For this review, take the finished solid that the model builds, in its own axes (mm). A direction names the side the tool comes from. Round coordinates to 2 decimals unless told otherwise and drop trailing zeros. Order: outer loops, then holes, each group sorted by start corner. A loop starts at its lowest first (then second) coordinate and runs counter-clockwise, first axis right, second up. Notation, with made-up numbers: (55, -12) -> (75, -12) arc R24 ccw to (75, 1) -> close; hole circle Ø1 at (85.25, 0). An arc over 180 degrees is marked (long way). Answer in a Markdown table with one row per item.
```python
from build123d import *

# Parameters (mm, degrees)
SKETCH_1_R               = 30
SKETCH_1_R_2             = 28.6
EXTRUDE_1_DEPTH          = 64
PATTERN_CIRCULAR_1_COUNT = 8
SKETCH_10_W              = 100
SKETCH_10_H              = 100
SKETCH_10_R              = 1.8
SKETCH_10_R_2            = 28.559863413
EXTRUDE_2_DEPTH          = 10


with BuildPart() as part:
    # 스케치1 → 보스-돌출1 (new body)
    with BuildSketch(Plane(origin=(0, 0, 0), x_dir=(1, 0, 0), z_dir=(0, 1, 0))):
        with Locations(Location((0, 0, 0), (0, 0, 270))):
            Circle(SKETCH_1_R)
        with Locations(Location((0, 0, 0), (0, 0, 270))):
            Circle(SKETCH_1_R_2, mode=Mode.SUBTRACT)
    extrude(amount=EXTRUDE_1_DEPTH)

    # 스케치9 → M2 남비 머리 나사용 카운터보어1 (revolve, cut)
    with BuildSketch(Plane(origin=(-30, 5, 0), x_dir=(0, 0, 1), z_dir=(0, 1, 0))):
        Polygon((0, 0), (0, 10.721032743), (1.2, 10), (1.2, 1), (2.5, 1), (2.5, 0), align=None)
    hole_wizard_m2_1 = revolve(axis=Axis((-36.35, 5, 0), (1, 0, 0)), mode=Mode.SUBTRACT)

    # 원형 패턴1: M2 남비 머리 나사용 카운터보어1 ×8 about axis
    pattern_circular_1_axis = Axis((0, 0, 0), (0, 1, 0))
    for i in range(1, PATTERN_CIRCULAR_1_COUNT):
        add(hole_wizard_m2_1.rotate(pattern_circular_1_axis, i * 360 / PATTERN_CIRCULAR_1_COUNT), mode=Mode.SUBTRACT)

    # 스케치10 → 보스-돌출2 (add)
    with BuildSketch(Plane(origin=(0, 64, 0), x_dir=(1, 0, 0), z_dir=(0, 1, 0))):
        Rectangle(SKETCH_10_W, SKETCH_10_H)
        with Locations(Location((41.7, -41.7, 0), (0, 0, 270))):
            Circle(SKETCH_10_R, mode=Mode.SUBTRACT)
        with Locations(Location((41.7, 41.7, 0), (0, 0, 270))):
            Circle(SKETCH_10_R, mode=Mode.SUBTRACT)
        with Locations(Location((-41.7, 41.7, 0), (0, 0, 270))):
            Circle(SKETCH_10_R, mode=Mode.SUBTRACT)
        with Locations(Location((-41.7, -41.7, 0), (0, 0, 270))):
            Circle(SKETCH_10_R, mode=Mode.SUBTRACT)
        with Locations(Location((0, 0, 0), (0, 0, 270))):
            Circle(SKETCH_10_R_2, mode=Mode.SUBTRACT)
    extrude(amount=EXTRUDE_2_DEPTH)


solid = part.part
```
Q1. Clearance check with flat-ended pins moving along their axes: pin 1 Ø4 at (x, y) = (0, 5) entering from +Z; pin 2 Ø4 at (x, y) = (0, 5) entering from -Z; pin 3 Ø2 at (x, y) = (-3, 13.5) entering from +Z; pin 4 Ø4.5 at (x, z) = (41.7, 41.7) entering from +Y. State where each tip first meets the part, or that it passes through.
Answer key:
| item | result |
|---|---|
| pin 1 | stops at z = 29 |
| pin 2 | stops at z = -29 |
| pin 3 | stops at z = 29.93 |
| pin 4 | stops at y = 74 |
Q2. Take a section at D-D, the plane x = -6.5. Write out the cut boundary in (y, z).
Answer key:
| item | result |
|---|---|
| outline | (0, -29.29) -> (64, -29.29) -> (64, -50) -> (74, -50) -> (74, -27.81) -> (64, -27.81) -> (64, -27.85) -> (0, -27.85) -> close; (0, 27.85) -> (64, 27.85) -> (64, 27.81) -> (74, 27.81) -> (74, 50) -> (64, 50) -> (64, 29.29) -> (0, 29.29) -> close |
Q3. Take a section at C-C, the plane z = -11.5. Write out the cut boundary in (x, y).
Answer key:
| item | result |
|---|---|
| outline | (-50, 64) -> (-27.71, 64) -> (-27.71, 0) -> (-26.19, 0) -> (-26.19, 64) -> (-26.14, 64) -> (-26.14, 74) -> (-50, 74) -> close; (26.14, 64) -> (26.19, 64) -> (26.19, 0) -> (27.71, 0) -> (27.71, 64) -> (50, 64) -> (50, 74) -> (26.14, 74) -> close |
Q4. Tool access review of faces 4 (the face through (-29, 4, -1)), 5 (the face through (-1, 6, -29)), 6 (the face through (22.55, 4.25, 19.18)), 7 (the face through (-11.49, 31.552, 27.712)), 8 (the face through (-1, 69, -50)): name each direction out of +Z, -Z, +X, -X, +Y, -Y from which nothing blocks a thin tool from reaching the whole face with its end or side.
Answer key:
| item | result |
|---|---|
| face 4 | -X |
| face 5 | -Z |
| face 6 | none |
| face 7 | -Y |
| face 8 | -Z, +X, -X, +Y, -Y |
Q5. To check wall thickness, follow probe 1 along X at (y, z) = (67.25, 0); probe 2 along Z at (x, y) = (0, 44.5); probe 3 along Z at (x, y) = (1, 3.5). State the ranges of each line that lie inside material, in increasing order.
Answer key:
| item | result |
|---|---|
| probe 1 | x = -50 to -28.56, 28.56 to 50 |
| probe 2 | z = -30 to -28.6, 28.6 to 30 |
| probe 3 | z = -29 to -28.58, 28.58 to 29 |
Q6. Take a section at A-A, the plane x = 41.7. Write out the cut boundary in (y, z), then the cut area to 3 significant figures.
Answer key:
| item | result |
|---|---|
| outline | (64, -50) -> (74, -50) -> (74, -43.5) -> (64, -43.5) -> close; (64, -39.9) -> (74, -39.9) -> (74, 39.9) -> (64, 39.9) -> close; (64, 43.5) -> (74, 43.5) -> (74, 50) -> (64, 50) -> close |
| area | 928 mm^2 |
Q7. Take a section at B-B, the plane z = -41.7. Write out the cut boundary in (x, y).
Answer key:
| item | result |
|---|---|
| outline | (-50, 64) -> (-43.5, 64) -> (-43.5, 74) -> (-50, 74) -> close; (-39.9, 64) -> (39.9, 64) -> (39.9, 74) -> (-39.9, 74) -> close; (43.5, 64) -> (50, 64) -> (50, 74) -> (43.5, 74) -> close |
Q8. The part is to be moulded in two halves that separate along Y. For faces 1 (the face through (-50, 69, 1)), 2 (the face through (-11, 0, 27)), 3 (the face through (-28.79, 3.99, 0.65)), say which applies: +Y half, -Y half, draft (parallel to the pull), parting line (faces both ways), or undercut.
Answer key:
| item | result |
|---|---|
| face 1 | draft |
| face 2 | -Y half |
| face 3 | undercut |
